```python
from build123d import *

# Parameters (mm, degrees)
BASE_EXTRUDE_DEPTH = 10


with BuildPart() as part:
    # Sketch1 → Base-Extrude (new body)
    with BuildSketch(Plane.XY):
        with BuildLine():
            Line((-24.513035081, -6.333333333), (-45.95357014, -6.333333333))
            Line((-45.95357014, -6.333333333), (-45.95357014, -1.333333333))
            Line((-45.95357014, -1.333333333), (-24.513035081, -1.333333333))
            ThreePointArc((-24.513035081, -1.333333333), (-18.739532389, 0.501700857), (-15.084944665, 5.333333333))
            ThreePointArc((-15.084944665, 5.333333333), (2.70563166, 15.769576954), (16, 0))
            Line((16, 0), (11, 0))
            ThreePointArc((11, 0), (1.860121766, 10.841584156), (-10.370899457, 3.666666667))
            ThreePointArc((-10.370899457, 3.666666667), (-15.852781043, -3.580782047), (-24.513035081, -6.333333333))
        make_face()
    extrude(amount=BASE_EXTRUDE_DEPTH)


solid = part.part
```
Model file for the job. Use its own axes, mm. A direction names the side the tool comes from. Round coordinates to 2 decimals unless told otherwise and drop trailing zeros. Write each loop counter-clockwise with the first axis right and the second up, starting at its lowest first coordinate (ties: lowest second). Pieces come first, ordered by that corner, then holes. Notation, with made-up numbers: M -11,-23 L 6,-23 A13 cw 6,-11 Z; hole C 29,-12 d1. An arc over 180 degrees is marked long. Put each result on its own line as item: value.
Item 1: Cut at D-D (y = 10). List the corners of the cut face in (x, z).
Responses:
outline: M -12.49,0 L -4.58,0 L -4.58,10 L -12.49,10 Z; M 4.58,0 L 12.49,0 L 12.49,10 L 4.58,10 Z
Item 2: Flat gauge pins, fed straight in: P1, Ø1.5, axis at x = -30, y = -1, coming from the -Z side; P2, Ø1, axis at y = 4, z = 5.5, coming from the +X side; P3, Ø1.5, axis at x = 14.5, z = 3, coming from the -Y side; P4, Ø4, axis at y = 13.5, z = 4, coming from the -X side. Where does each tip first touch, or does it go through?
Responses:
P1: z = 0
P2: x = 15.61
P3: y = 0
P4: x = -11.12
Item 3: Mould opens along X. For faces 1 (the cylindrical face through (-15.748, -3.506, 4.93)), 2 (the flat face through (-45.954, -4, 5)), 3 (the flat face through (-35, -1.333, 5)) say: +X half, -X half, draft (parallel to the pull), parting line (faces both ways), or undercut.
Responses:
face 1: undercut
face 2: -X half
face 3: draft
Item 4: Probe L1, parallel to Y at x = 0.5, z = 2.5; L2, parallel to Y at x = -37, z = 6.5; L3, parallel to X at y = 4.5, z = 3.75. List the from-to ranges inside material, lowest first. Write a range as from..to.
Responses:
L1: 10.99..15.99
L2: -6.33..-1.33
L3: -15.42..-10.04, 10.04..15.35
Item 5: Tool access for faces 4 (the flat face through (14, 0, 5)), 5 (the cylindrical face through (2.4, 15.82, 4.93)): list every direction of +Z, -Z, +X, -X, +Y, -Y with a clear straight run to the whole face (end or side of a thin tool).
Responses:
face 4: +Z, -Z, +X, -Y
face 5: +Z, -Z, +Y
Item 6: Cut at C-C (x = -39.5). List the corners of the cut face in (y, z).
Responses:
outline: M -6.33,0 L -1.33,0 L -1.33,10 L -6.33,10 Z
Item 7: Cut at A-A (z = 2). List the corners of the cut face in (x, y), and give its area (3 significant figures).
Responses:
outline: M -45.95,-6.33 L -24.51,-6.33 A15 ccw -10.37,3.67 A11 cw 11,0 L 16,0 A16 ccw -15.08,5.33 A10 cw -24.51,-1.33 L -45.95,-1.33 Z
area: 373 mm²
Item 8: Cut at B-B (y = 1.5). List the corners of the cut face in (x, z), and give its area (3 significant figures).
Responses:
outline: M -17.54,0 L -11.34,0 L -11.34,10 L -17.54,10 Z; M 10.9,0 L 15.93,0 L 15.93,10 L 10.9,10 Z
area: 112 mm²
